Check sheet for the drawn part. Datum: minimum x, y, z corner. Units: mm. Give positions to 0.01 mm unless a question says otherwise; leave off trailing zeros. Write each loop counter-clockwise with the first axis right and the second up, starting at its lowest first coordinate (ties: lowest second). Pieces come first, ordered by that corner, then holes. Notation, with made-up numbers: (-26.5, 70) - (-22.5, 70) arc R17 ccw to (-22.5, 89) - close; hole circle Ø1 at (44.25, 31.5). An arc over 180 degrees is marked (long way). Answer as a JSON object with one key per item and string values. Group by question number.
Item 1: Go/stop test with a flat-tipped pin: pin 1 (1.5 mm diameter, centred on y = 39.5, z = 1, fed in from -X). Record where the tip stops, or that it passes through.
Item 2: Sectioned sample at A-A, the plane z = 1.3. Record the boundary of the cut face in (x, y), and give its area (3 significant figures).
Item 3: Scan line: line 1 along X through (y, z) = (16, 0.3). Record every from-to range of solid material in increasing order. Write a range as [from, to].
Item 4: Sectioned sample at B-B, the plane y = 12.5. Record the boundary of the cut face in (x, z), and give its area (3 significant figures).
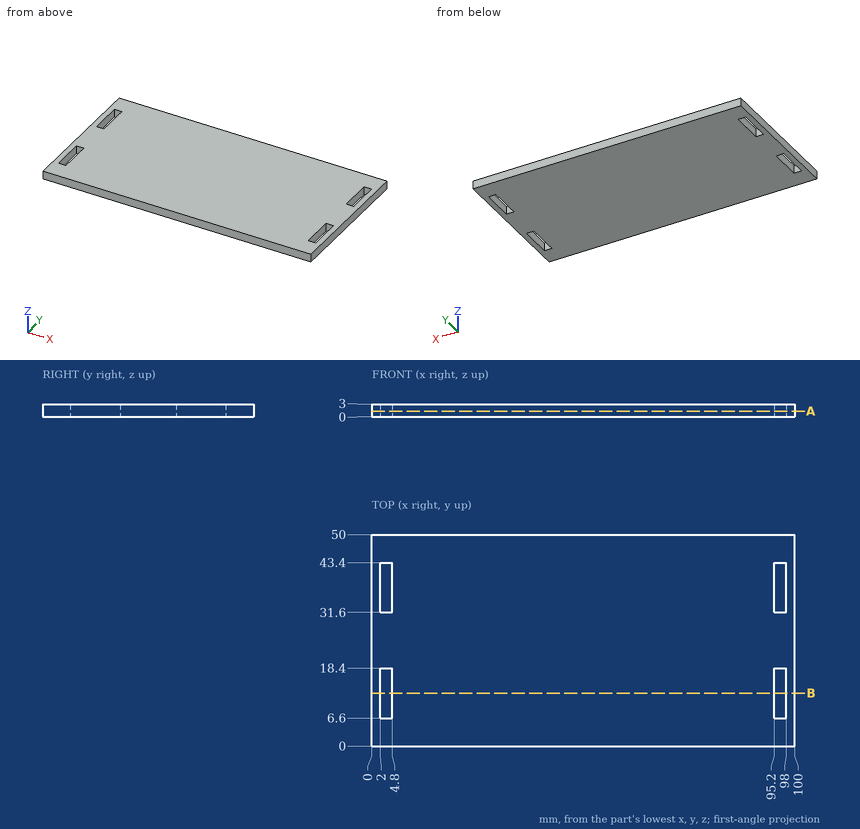
Geometry check:
{
 "1": {"pin 1": "x = 0"},
 "2": {"outline": "(0, 0) - (100, 0) - (100, 50) - (0, 50) - close; hole (2, 6.6) - (4.8, 6.6) - (4.8, 18.4) - (2, 18.4) - close; hole (2, 31.6) - (4.8, 31.6) - (4.8, 43.4) - (2, 43.4) - close; hole (95.2, 6.6) - (98, 6.6) - (98, 18.4) - (95.2, 18.4) - close; hole (95.2, 31.6) - (98, 31.6) - (98, 43.4) - (95.2, 43.4) - close", "area": "4,870 mm^2"},
 "3": {"line 1": "[0, 2], [4.8, 95.2], [98, 100]"},
 "4": {"outline": "(0, 0) - (2, 0) - (2, 3) - (0, 3) - close; (4.8, 0) - (95.2, 0) - (95.2, 3) - (4.8, 3) - close; (98, 0) - (100, 0) - (100, 3) - (98, 3) - close", "area": "283 mm^2"}
}
